from build123d import *

# Parameters (mm, degrees)
BOSS_EXTRUDE2_DEPTH          = 482.6
CUT_EXTRUDE3_DEPTH           = 488.592555637
SKETCH7_R                    = 7.9629
CUT_EXTRUDE4_DEPTH           = 488.592555637
F_10_0_1935_DIAMETER_HOLE1_D = 4.999999906


with BuildPart() as part:
    # Sketch3 → Boss-Extrude2 (new body)
    with BuildSketch(Plane.XY):
        Polygon((0, 0), (0, 49.2125), (-1.5875, 49.2125), (-1.5875, -1.5875), (49.2125, -1.5875), (49.2125, 0), align=None)
    extrude(amount=BOSS_EXTRUDE2_DEPTH)

    # Sketch6 → Cut-Extrude3 (cut, through all)
    with BuildSketch(Plane(origin=(0, 0, 0), x_dir=(0, 0, -1), z_dir=(1, 0, 0))):
        with BuildLine():
            Line((-434.848, 39.1795), (-231.648, 39.1795))
            ThreePointArc((-231.648, 39.1795), (-217.297, 24.8285), (-231.648, 10.4775))
            Line((-231.648, 10.4775), (-434.848, 10.4775))
            ThreePointArc((-434.848, 10.4775), (-449.199, 24.8285), (-434.848, 39.1795))
        make_face()
    extrude(amount=-CUT_EXTRUDE3_DEPTH, mode=Mode.SUBTRACT)

    # Sketch7 → Cut-Extrude4 (cut, through all)
    with BuildSketch(Plane(origin=(0, 0, 0), x_dir=(0, 0, -1), z_dir=(1, 0, 0))):
        with Locations(Location((-80.264, 24.773594829, 0), (0, 0, 90))):
            Circle(SKETCH7_R)
    extrude(amount=-CUT_EXTRUDE4_DEPTH, mode=Mode.SUBTRACT)

    # #10 (0.1935) Diameter Hole1 (through all)
    with Locations(Plane(origin=(0, 0, 0), x_dir=(0, 0, -1), z_dir=(1, 0, 0))):
        with Locations((-434.848, 43.2435), (-384.048, 43.2435), (-333.248, 43.2435), (-282.448, 43.2435), (-231.648, 43.2435), (-231.648, 6.4135), (-282.448, 6.4135), (-333.248, 6.4135), (-384.048, 6.4135), (-434.848, 6.4135)):
            Hole(F_10_0_1935_DIAMETER_HOLE1_D / 2)


solid = part.part
Geometry: final body of the model. Coordinates: model frame, mm. A direction names the side the tool comes from. Give positions to 0.01 mm unless a question says otherwise; leave off trailing zeros. Order: outer loops, then holes, each group sorted by start corner. A loop starts at its lowest first (then second) coordinate and runs counter-clockwise, first axis right, second up. Notation, with made-up numbers: (61, -27) -> (69, -27) arc R33 cw to (69, 6) -> close; hole circle Ø1 at (51, 32.5). An arc over 180 degrees is marked (long way). Put each result on its own line as item: value.
Q1. Section D-D, the plane x = 19. Return loops of the section in (y, z).
Here are the results:
outline: (-1.59, 0) -> (0, 0) -> (0, 482.6) -> (-1.59, 482.6) -> close
Q2. Pin query (flat end, axial travel): pin 1 (15 mm diameter, centred on x = 23, z = 283, fed in from +Y); pin 2 (5.5 mm diameter, centred on y = 6.41, z = 231.65, fed in from +X). Return the tip coordinate at first contact, or that it passes through.
Here are the results:
pin 1: stops at y = 0
pin 2: stops at x = 0
Q3. Draft query along Z for faces 1 (the face through (-1, 13, 0)), 2 (the face through (-0.8, 25.1, 217.3)), 3 (the face through (25, 0, 238)). Return one class per face: released by +Z, released by -Z, zero draft, split by the parting line, or undercut.
Here are the results:
face 1: released by -Z
face 2: undercut
face 3: zero draft
Q4. Section C-C, the plane z = 194.5. Return loops of the section in (x, y), then the cut area to 3 significant figures.
Here are the results:
outline: (-1.59, -1.59) -> (49.21, -1.59) -> (49.21, 0) -> (0, 0) -> (0, 49.21) -> (-1.59, 49.21) -> close
area: 159 mm^2
Q5. Section B-B, the plane y = 26. Return loops of the section in (x, z), then the cut area to 3 significant figures.
Here are the results:
outline: (-1.59, 0) -> (0, 0) -> (0, 72.4) -> (-1.59, 72.4) -> close; (-1.59, 88.13) -> (0, 88.13) -> (0, 217.34) -> (-1.59, 217.34) -> close; (-1.59, 449.15) -> (0, 449.15) -> (0, 482.6) -> (-1.59, 482.6) -> close
area: 373 mm^2
Q6. Section A-A, the plane z = 357.5. Return loops of the section in (x, y).
Here are the results:
outline: (-1.59, -1.59) -> (49.21, -1.59) -> (49.21, 0) -> (0, 0) -> (0, 10.48) -> (-1.59, 10.48) -> close; (-1.59, 39.18) -> (0, 39.18) -> (0, 49.21) -> (-1.59, 49.21) -> close
Q7. Reachability of faces 4 (the face through (-1.588, 41, 238)), 5 (the face through (-0.783, 24.513, 449.196)), 6 (the face through (0, 41, 238)) from +Z, -Z, +X, -X, +Y, -Y: full face, straight path, thin tool, end or side. Return the list, or none.
Here are the results:
face 4: +Z, -Z, -X, +Y, -Y
face 5: +X, -X
face 6: +Z, -Z, +X, +Y
Q8. Material intervals for L1, parallel to X at y = 42, z = 99.5, sorted ascending.
Here are the results:
L1: x = -1.59 to 0
